Check sheet for the drawn part. Datum: minimum x, y, z corner. Units: mm. Coordinates: 2 decimals unless noted, no trailing zeros. Write each loop counter-clockwise with the first axis right and the second up, starting at its lowest first coordinate (ties: lowest second). Pieces come first, ordered by that corner, then holes. Notation, with made-up numbers: (-3, 88.25) -> (39, 88.25) arc R31 ccw to (39, 121.25) -> close; hole circle Ø10 at (18, -18). An arc over 180 degrees is marked (long way). Answer in a Markdown table with one row per item. Add a question column.
1. Cross-section at A-A on y = 61.5. Record the cut outline in (x, z).
2. Cross-section at C-C on y = 28.5. Record the cut outline in (x, z).
3. Depth check by flat-ended pin: P1, Ø1.2, axis at x = 54, z = 20, coming from the -Y side; P2, Ø0.8, axis at y = 62, z = 20, coming from the -X side; P3, Ø0.8, axis at y = 60.5, z = 19.5, coming from the +X side. Enter the tip coordinate at first touch or a pass-through.
4. Scan lines: L1, parallel to Z at x = 20.5, y = 50.5; L2, parallel to X at y = 58, z = 1.75; L3, parallel to X at y = 11, z = 18. Record each from-to range of solid material in increasing order. Write a range as from..to.
5. Cross-section at B-B on x = 59. Record the cut outline in (y, z).
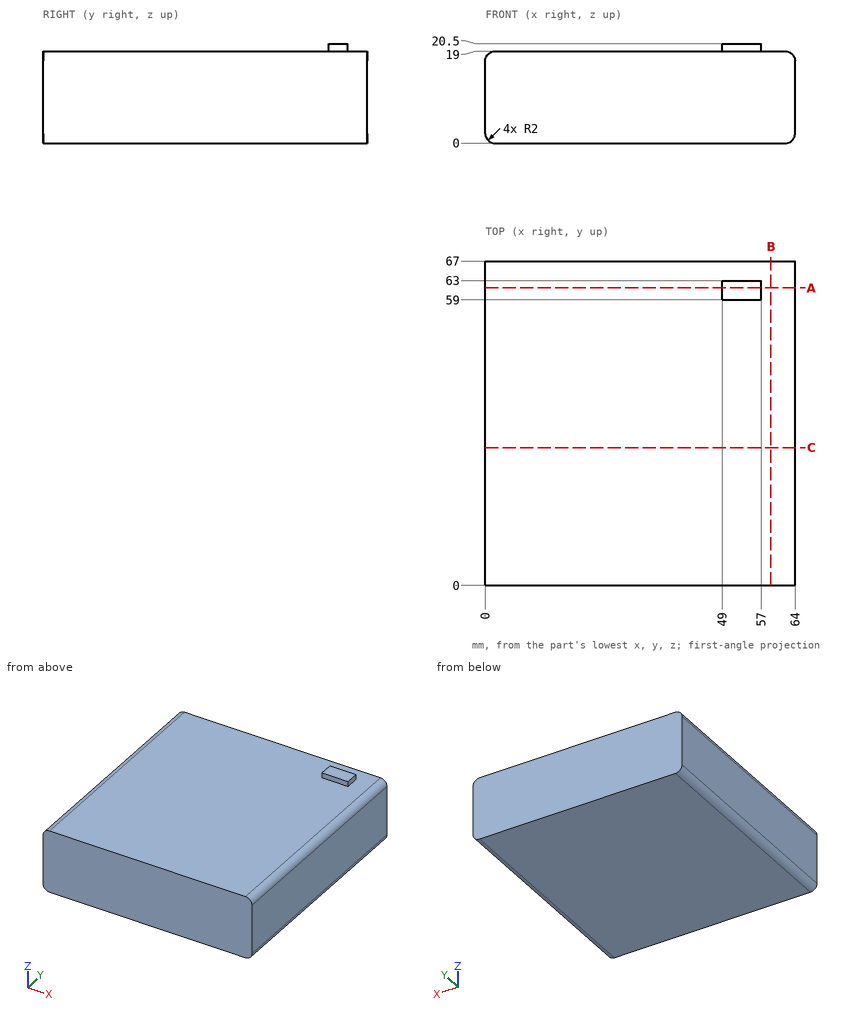
Results found:
| question | item | result |
|---|---|---|
| 1 | outline | (0, 2) arc R2 ccw to (2, 0) -> (62, 0) arc R2 ccw to (64, 2) -> (64, 17) arc R2 ccw to (62, 19) -> (57, 19) -> (57, 20.5) -> (49, 20.5) -> (49, 19) -> (2, 19) arc R2 ccw to (0, 17) -> close |
| 2 | outline | (0, 2) arc R2 ccw to (2, 0) -> (62, 0) arc R2 ccw to (64, 2) -> (64, 17) arc R2 ccw to (62, 19) -> (2, 19) arc R2 ccw to (0, 17) -> close |
| 3 | P1 | stops at y = 59 |
| 3 | P2 | stops at x = 49 |
| 3 | P3 | stops at x = 57 |
| 4 | L1 | z = 0..19 |
| 4 | L2 | x = 0.02..63.98 |
| 4 | L3 | x = 0.27..63.73 |
| 5 | outline | (0, 0) -> (67, 0) -> (67, 19) -> (0, 19) -> close |
